Could you check a few things on this model? Use its own coordinates, in mm. A direction names the side the tool comes from. Give positions to 0.01 mm unless a question says otherwise; leave off trailing zeros. Write each loop counter-clockwise with the first axis right and the second up, starting at its lowest first coordinate (ties: lowest second). Pieces come first, ordered by that corner, then holes. Notation, with made-up numbers: (32.25, 9) - (71.25, 9) arc R30 ccw to (71.25, 37) - close; hole circle Ø7 at (2.5, 38). An arc over 180 degrees is marked (long way). Answer in a Markdown table with one row per item.
Autodesk Inventor part; units mm, degrees
ref_plane "Pracovní rovina11" through (0, 0, 164) normal (0, 0, 1) x (1, 0, 0)
ref_plane "YZ Plane" through (0, 0, 0) normal (1, 0, 0) x (0, 1, 0)
ref_plane "XZ Plane" through (0, 0, 0) normal (0, 1, 0) x (-1, 0, 0)
ref_plane "Pracovní rovina11" through (0, 0, 164) normal (0, 0, 1) x (1, 0, 0)
sketch "Náčrt11" plane through (0, 0, 164) normal (0, 0, 1) x (1, 0, 0)
  line L0 (-0.5, -50.5) -> (190.5, -50.5)
  line L1 (190.5, -50.5) -> (190.5, 0.5)
  line L2 (190.5, 0.5) -> (-0.5, 0.5)
  line L3 (-0.5, 0.5) -> (-0.5, -50.5)
  line L4 (0, 0) -> (0, -50)
  line L5 (190, -50) -> (190, 0)
  line L6 (190, 0) -> (0, 0)
  line L7 (182, -50) -> (58, -50)
  line L8 (-4.5, 4.5) -> (194.5, 4.5)
  line L9 (194.5, 4.5) -> (194.5, -54.5)
  line L10 (194.5, -54.5) -> (-4.5, -54.5)
  line L11 (-4.5, -54.5) -> (-4.5, 4.5)
  dimension "d43" = 0.5
  dimension "d44" = 0.5
  dimension "d45" = 0.5
  dimension "d46" = 0.5
  dimension "d47" = 4
extrude "Vysunutí11" add sketch "Náčrt11" against normal blind 8
sketch "Náčrt12" plane through (0, 0, 164) normal (0, 0, 1) x (1, 0, 0)
  line L0 (-4.5, 4.5) -> (-4.5, -54.5)
  line L1 (194.5, 4.5) -> (-4.5, 4.5)
  line L2 (194.5, -54.5) -> (194.5, 4.5)
  line L3 (-4.5, -54.5) -> (194.5, -54.5)
  point P0 (0, 0)
extrude "Vysunutí12" add sketch "Náčrt12" along normal blind 4
sketch "Náčrt13" plane through (0, 0, 168) normal (0, 0, 1) x (1, 0, 0)
  circle A0 centre (5.5, -25) radius 2.5
  circle A1 centre (184.5, -25) radius 2.5
  line L0 (-4.5, -54.5) -> (194.5, -54.5)
  line L1 (194.5, 4.5) -> (-4.5, 4.5)
  line L2 (-4.5, 4.5) -> (-4.5, -54.5)
  line L3 (194.5, -54.5) -> (194.5, 4.5)
  point P0 (0, 0)
  dimension "d52" = 5
  dimension "d53" = 5
  dimension "d54" = 59
  dimension "d55" = 29.5
  dimension "d56" = 29.5
  dimension "d57" = 10
  dimension "d58" = 10
extrude "Vysunutí13" cut sketch "Náčrt13" against normal through all contours A0 | A1
sketch "Náčrt14" plane through (-4.5, 4.5, 156) normal (0, 1, 0) x (1, 0, 0)
  line L0 (4, -8) -> (4, 0)
  line L1 (195, -8) -> (195, 0)
  line L2 (4, -8) -> (195, -8)
  line L3 (0, 0) -> (199, 0)
  point P0 (4.5, 156)
extrude "Vysunutí14" cut sketch "Náčrt14" against normal up to surface (4 mm away)
sketch "Náčrt15" plane through (-4.5, 4.5, 168) normal (0, 1, 0) x (1, 0, 0)
  line L0 (199, 0) -> (0, 0)
  line L1 (199, 12) -> (199, 0)
  line L2 (195, 12) -> (195, 4)
  line L3 (195, 4) -> (4, 4)
  line L4 (4, 4) -> (4, 12)
  line L5 (0, 12) -> (0, 0)
  line L6 (0, 12) -> (4, 12)
  line L7 (195, 12) -> (199, 12)
  point P0 (4.5, 168)
extrude "Vysunutí15" cut sketch "Náčrt15" against normal blind 5
properties part number "krab1-ver1" material "11 500"
1) If I drill on line 1 (Y direction, x = 5.5, z = 166.3); line 2 (X direction, y = -6.5, z = 156.5); line 3 (Z direction, x = 40.5, y = -33), over which ranges is the centre line in solid material (lowest first)?
Check values:
| item | result |
|---|---|
| line 1 | y = -54.5 to -27.5, -22.5 to -0.5 |
| line 2 | x = -4.5 to -0.5, 190.5 to 194.5 |
| line 3 | z = 164 to 168 |
2) Imagine slicing it at D-D (z = 158). List the corners of the cut face in (x, y) for me.
Check values:
| item | result |
|---|---|
| outline | (-4.5, -54.5) - (194.5, -54.5) - (194.5, -0.5) - (190.5, -0.5) - (190.5, -50.5) - (-0.5, -50.5) - (-0.5, -0.5) - (-4.5, -0.5) - close |
3) Imagine slicing it at C-C (y = -11). List the corners of the cut face in (x, z) for me, then the cut area to 3 significant figures.
Check values:
| item | result |
|---|---|
| outline | (-4.5, 156) - (-0.5, 156) - (-0.5, 164) - (190.5, 164) - (190.5, 156) - (194.5, 156) - (194.5, 168) - (-4.5, 168) - close |
| area | 860 mm2 |
4) We'd pull the mould along Y, two halves only. Please class faces 1 (the face through (87, -0.5, 166)), 2 (the face through (186.885, -24.249, 166.028)), 3 (the face through (94, -27, 168)), 4 (the face through (7, -23, 166)): +Y half, -Y half, draft (parallel to the pull), parting line (faces both ways), or undercut.
Check values:
| item | result |
|---|---|
| face 1 | +Y half |
| face 2 | undercut |
| face 3 | draft |
| face 4 | undercut |
5) Imagine slicing it at A-A (x = 184.5). List the corners of the cut face in (y, z) for me, then the cut area to 3 significant figures.
Check values:
| item | result |
|---|---|
| outline | (-54.5, 156) - (-50.5, 156) - (-50.5, 164) - (-27.5, 164) - (-27.5, 168) - (-54.5, 168) - close; (-22.5, 164) - (-0.5, 164) - (-0.5, 168) - (-22.5, 168) - close |
| area | 228 mm2 |
6) On a 3-axis mill with a long thin cutter (end or side, diameter ignored), from which of +Z, -Z, +X, -X, +Y, -Y can I reach the whole of each face in a straight line? I mean faces 5 (the face through (65, -51, 156)), 6 (the face through (-0.5, -25, 160)). Say none if no direction works.
Check values:
| item | result |
|---|---|
| face 5 | -Z, +X, -X, +Y, -Y |
| face 6 | -Z, +Y |
7) Imagine slicing it at B-B (y = -25). List the corners of the cut face in (x, z) for me, then the cut area to 3 significant figures.
Check values:
| item | result |
|---|---|
| outline | (-4.5, 156) - (-0.5, 156) - (-0.5, 164) - (3, 164) - (3, 168) - (-4.5, 168) - close; (8, 164) - (182, 164) - (182, 168) - (8, 168) - close; (187, 164) - (190.5, 164) - (190.5, 156) - (194.5, 156) - (194.5, 168) - (187, 168) - close |
| area | 820 mm2 |
8) Will these pins go through, and if not, where does the flat tip stop? P1, Ø5, axis at x = 134, z = 157.5, coming from the +Y side; P2, Ø3, axis at x = 184.5, y = -25, coming from the +Z side; P3, Ø5, axis at x = 96.5, y = -23.5, coming from the -Z side.
Check values:
| item | result |
|---|---|
| P1 | stops at y = -50.5 |
| P2 | passes through |
| P3 | stops at z = 164 |
